Part model, mm, in its own coordinate system. A direction names the side the tool comes from. Round coordinates to 2 decimals unless told otherwise and drop trailing zeros. Loops run counter-clockwise (first coordinate to the right, second up) from the corner with the lowest first, then second, coordinate; pieces in that order, holes last.
(1) Mould opens along Z. For faces 1 (the face through (0, 26, 5.08)), 2 (the face through (21.346, -35.828, 3.263)), 3 (the face through (0.69, -3.1, 5.01)) say: +Z half, -Z half, draft (parallel to the pull), parting line (faces both ways), or undercut.
(2) Flat gauge pins, fed straight in: pin 1 (5 mm diameter, centred on y = 27, z = 8, fed in from +X); pin 2 (5 mm diameter, centred on y = 0, z = 5.08, fed in from -X); pin 3 (5 mm diameter, centred on x = 0, y = 0, fed in from -Z); pin 4 (5 mm diameter, centred on x = -1.5, y = 12.5, fed in from +Z). Where does each tip first touch, or does it go through?
(3) Tool access for faces 4 (the face through (41.7, -0.73, 3.32)), 5 (the face through (-0.07, 40.6, 7.58)), 6 (the face through (-19.027, -33.009, 5.107)): list every direction of +Z, -Z, +X, -X, +Y, -Y with a clear straight run to the whole face (end or side of a thin tool).
(4) Cut at A-A on y = 0. List the corners of the cut face in (x, z) (1 decimal).
(5) Probe probe 1 along Y at (x, z) = (0, 5.75) (1 decimal); probe 2 along Y at (x, z) = (0, 3.75) (1 decimal); probe 3 along X at (y, z) = (-35.5, 4). List the from-to ranges inside material, lowest first.
from build123d import *

# Parameters (mm, degrees)
SKETCH1_R           = 45.4025
BOSS_EXTRUDE1_DEPTH = 10.16
CUT_EXTRUDE1_START  = 38.1
SKETCH2_R           = 1.905
CUT_EXTRUDE1_DEPTH  = 7.62
CIRPATTERN1_COUNT   = 6
SKETCH3_R           = 3.175
CUT_EXTRUDE2_DEPTH  = 66.007689034
CUT_EXTRUDE3_DEPTH  = 5.08
CHAMFER2_SIZE       = 5.08


with BuildPart() as part:
    # Sketch1 → Boss-Extrude1 (new body)
    with BuildSketch(Plane.XY):
        Circle(SKETCH1_R)
    extrude(amount=BOSS_EXTRUDE1_DEPTH)

    # Sketch2 → Cut-Extrude1 (cut)
    with BuildSketch(Plane(origin=(0, 0, 0), x_dir=(0, 0, -1), z_dir=(1, 0, 0)).offset(CUT_EXTRUDE1_START)):
        with Locations((-5.08, 0)):
            Circle(SKETCH2_R)
    cut_extrude1 = extrude(amount=CUT_EXTRUDE1_DEPTH, mode=Mode.SUBTRACT)

    # CirPattern1: Cut-Extrude1 ×6 about axis
    cirpattern1_axis = Axis((0, 0, 0), (0, 0, 1))
    for i in range(1, CIRPATTERN1_COUNT):
        add(cut_extrude1.rotate(cirpattern1_axis, i * 360 / CIRPATTERN1_COUNT), mode=Mode.SUBTRACT)

    # Sketch3 → Cut-Extrude2 (cut, through all)
    with BuildSketch(Plane(origin=(0, 0, 0), x_dir=(-1, 0, 0), z_dir=(0, 0, -1))):
        Circle(SKETCH3_R)
    extrude(amount=-CUT_EXTRUDE2_DEPTH, mode=Mode.SUBTRACT)

    # Sketch4 → Cut-Extrude3 (cut)
    with BuildSketch(Plane.XY.offset(10.16)):
        with BuildLine():
            Line((-5.08, 38.1), (5.08, 38.1))
            ThreePointArc((5.08, 38.1), (6.876051224, 37.356051224), (7.62, 35.56))
            Line((7.62, 35.56), (7.62, 15.24))
            ThreePointArc((7.62, 15.24), (6.876051224, 13.443948776), (5.08, 12.7))
            Line((5.08, 12.7), (-5.08, 12.7))
            ThreePointArc((-5.08, 12.7), (-6.876051224, 13.443948776), (-7.62, 15.24))
            Line((-7.62, 15.24), (-7.62, 35.56))
            ThreePointArc((-7.62, 35.56), (-6.876051224, 37.356051224), (-5.08, 38.1))
        make_face()
    extrude(amount=-CUT_EXTRUDE3_DEPTH, mode=Mode.SUBTRACT)

    # Chamfer2
    chamfer2_edges = [part.edges().sort_by_distance(p)[0] for p in [
        (0, 12.7, 10.16),
        (6.876051224, 13.443948776, 10.16),
        (-6.876051224, 13.443948776, 10.16),
        (7.62, 25.4, 10.16),
        (-7.62, 25.4, 10.16),
        (6.876051224, 37.356051224, 10.16),
        (-6.876051224, 37.356051224, 10.16),
        (0, 38.1, 10.16),
    ]]
    chamfer(chamfer2_edges, length=CHAMFER2_SIZE - 0.0001)  # a hair under: the kernel refuses the full size


solid = part.part
Final values:
1. face 1: +Z half
1. face 2: undercut
1. face 3: draft
2. pin 1: stops at x = 38.22
2. pin 2: stops at x = -45.4
2. pin 3: passes through
2. pin 4: stops at z = 7.78
3. face 4: +X
3. face 5: +Z
3. face 6: none
4. outline: (-45.4, 0) - (-3.2, 0) - (-3.2, 10.2) - (-45.4, 10.2) - (-45.4, 7) - (-38.1, 7) - (-38.1, 3.2) - (-45.4, 3.2) - close; (3.2, 0) - (45.4, 0) - (45.4, 3.2) - (38.1, 3.2) - (38.1, 7) - (45.4, 7) - (45.4, 10.2) - (3.2, 10.2) - close
5. probe 1: y = -45.4 to -3.2, 3.2 to 12, 38.8 to 45.4
5. probe 2: y = -45.4 to -3.2, 3.2 to 45.4
5. probe 3: x = -28.3 to -22.31, -18.68 to 18.68, 22.31 to 28.3
